Geometry: see drawing. Coordinates: mm, zero at the bounding-box minimum. A direction names the side the tool comes from. Give positions to 0.01 mm unless a question says otherwise; leave off trailing zeros. Order: outer loops, then holes, each group sorted by start corner. A loop starts at its lowest first (then second) coordinate and runs counter-clockwise, first axis right, second up. Notation, with made-up numbers: M 21.25,-6 L 43.25,-6 A9 cw 43.25,0 Z; hole C -20,10 d4. An arc over 180 degrees is marked long. Use a Markdown table: item, result.
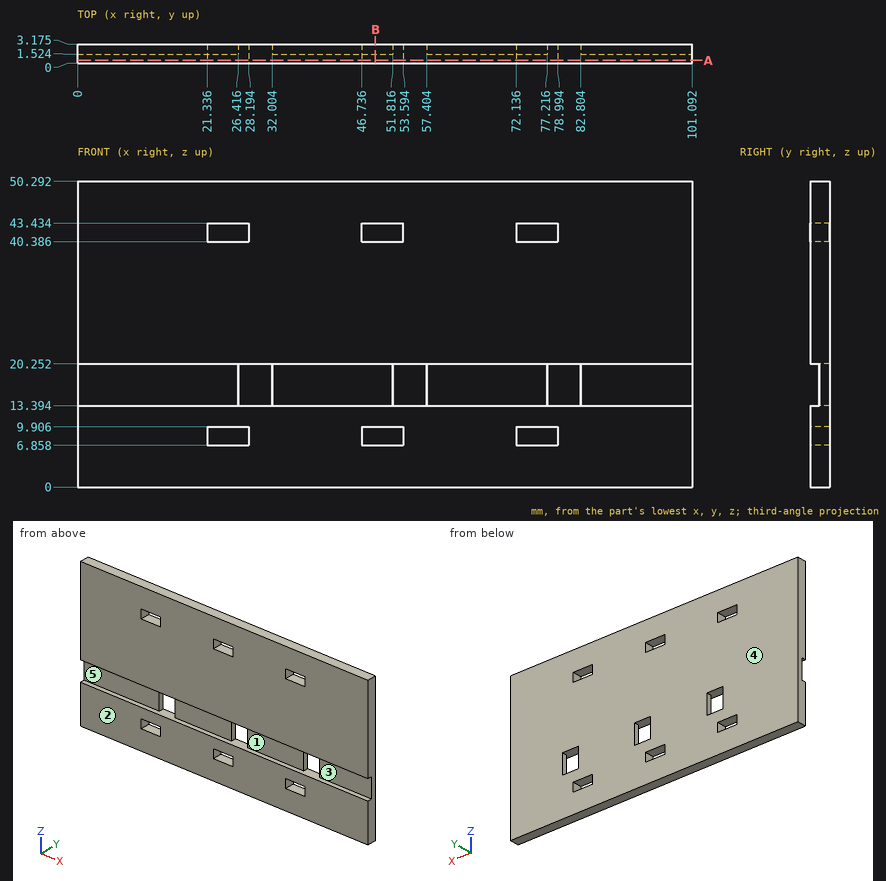
1) First-contact query: pin 1 Ø3.5 at (x, z) = (43.5, 16.5) entering from -Y. Flat tip, straight axial feed; report the tip coordinate or a pass-through.
Response values:
| item | result |
|---|---|
| pin 1 | stops at y = 1.52 |
2) Reachability of the marked faces 1 and 2 from +Z, -Z, +X, -X, +Y, -Y: full face, straight path, thin tool, end or side. Return the list, or none.
Response values:
| item | result |
|---|---|
| face 1 | +X, -X, -Y |
| face 2 | +Z, -Z, +X, -X, -Y |
3) Cut plane B-B on x = 49. Return loops of the section in (y, z) (1 decimal), and give its area (3 significant figures).
Response values:
| item | result |
|---|---|
| outline | M 0,0 L 3.2,0 L 3.2,6.9 L 0,6.9 Z; M 0,9.9 L 3.2,9.9 L 3.2,40.4 L 0,40.4 L 0,20.3 L 1.5,20.3 L 1.5,13.4 L 0,13.4 Z; M 0,43.4 L 3.2,43.4 L 3.2,50.3 L 0,50.3 Z |
| area | 130 mm² |
4) Cut plane A-A on y = 0.5. State how many separate pieces and enclosed holes the cut face has.
Response values:
| item | result |
|---|---|
| separate pieces | 2 |
| enclosed holes | 6 |
5) Mould query, pull axis Z, two halves, no side actions, for the marked faces 3, 4 and 5. Classes: released by +Z, released by -Z, zero draft, split by the parting line, or undercut.
Response values:
| item | result |
|---|---|
| face 3 | undercut |
| face 4 | zero draft |
| face 5 | undercut |
6) Material intervals for line 1 (X direction, y = 2.25, z = 42.5); line 2 (Z direction, x = 76.5, y = 0.45) (1 decimal); line 3 (X direction, y = 2.2, z = 16), sorted ascending. Write a range as from..to.
Response values:
| item | result |
|---|---|
| line 1 | x = 0..21.34, 28.19..46.74, 53.59..72.14, 78.99..101.09 |
| line 2 | z = 0..6.9, 9.9..13.4, 20.3..40.4, 43.4..50.3 |
| line 3 | x = 0..26.42, 32..51.82, 57.4..77.22, 82.8..101.09 |
